Geometry check sheet. Reference: drawing and pictorial views, mm from the part's lowest x, y, z. A direction names the side the tool comes from. Coordinates: 2 decimals unless noted, no trailing zeros. Order: outer loops, then holes, each group sorted by start corner. A loop starts at its lowest first (then second) coordinate and runs counter-clockwise, first axis right, second up. Notation, with made-up numbers: M 78.25,20 L 84.25,20 A21 cw 84.25,30 Z; hole C 79.5,16.5 d10. An arc over 180 degrees is marked long. Return JSON: item names as keys, results as strings.
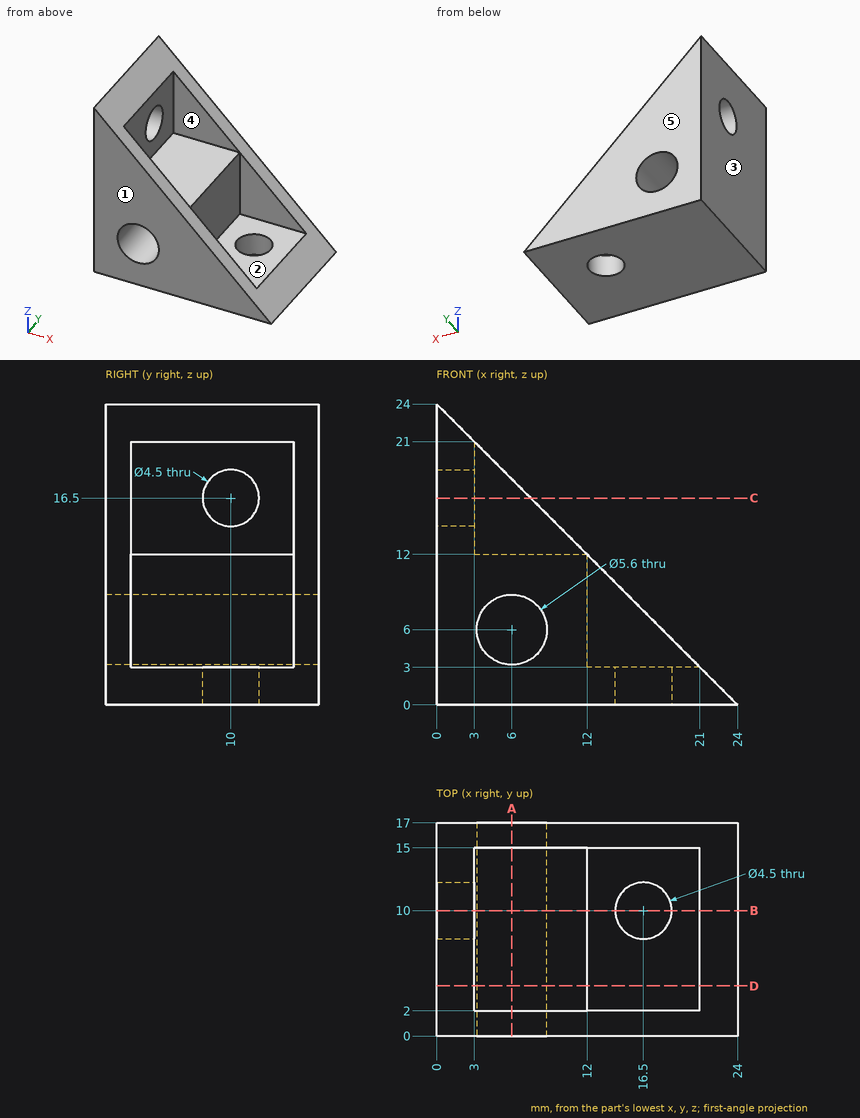
Q1. Cross-section at C-C, the plane z = 16.5. Record the boundary of the cut face in (x, y), and give its area (3 significant figures).
Values:
{"outline": "M 0,0 L 7.5,0 L 7.5,2 L 3,2 L 3,7.75 L 0,7.75 Z; M 0,12.25 L 3,12.25 L 3,15 L 7.5,15 L 7.5,17 L 0,17 Z", "area": "55.5 mm^2"}
Q2. Material ranges on line 1 along Y through (x, z) = (4, 15.5); line 2 along Y through (x, z) = (16.5, 1.4); line 3 along Z through (x, y) = (6, 5.25), recorded low to high.
Values:
{"line 1": "0 to 2, 15 to 17", "line 2": "0 to 7.75, 12.25 to 17", "line 3": "0 to 3.2, 8.8 to 12"}
Q3. Cross-section at D-D, the plane y = 4. Record the boundary of the cut face in (x, z), and give its area (3 significant figures).
Values:
{"outline": "M 0,0 L 24,0 L 21,3 L 12,3 L 12,12 L 3,12 L 3,21 L 0,24 Z; hole C 6,6 d5.6", "area": "182 mm^2"}
Q4. Cross-section at A-A, the plane x = 6. Record the boundary of the cut face in (y, z), and give its area (3 significant figures).
Values:
{"outline": "M 0,0 L 17,0 L 17,3.2 L 0,3.2 Z; M 0,8.8 L 17,8.8 L 17,18 L 15,18 L 15,12 L 2,12 L 2,18 L 0,18 Z", "area": "133 mm^2"}
Q5. Go/stop test with flat-tipped pins: pin 1 (2.5 mm diameter, centred on x = 17.5, y = 8.5, fed in from +Z); pin 2 (7 mm diameter, centred on y = 10, z = 16.5, fed in from -X); pin 3 (2 mm diameter, centred on y = 5, z = 16, fed in from +X); pin 4 (2.5 mm diameter, centred on x = 9.5, y = 9, fed in from +Z). Record where each tip stops, or that it passes through.
Values:
{"pin 1": "z = 3", "pin 2": "x = 0", "pin 3": "x = 3", "pin 4": "z = 12"}
Q6. Tool access check on the marked faces 4 and 5. Record the directions out of +Z, -Z, +X, -X, +Y, -Y that give a thin tool (end or side, any length) a straight path to the whole face; none if there is none.
Values:
{"face 4": "+Z, +X", "face 5": "+Z, -Z, +X, -X, +Y"}
Q7. Cross-section at B-B, the plane y = 10. Record the boundary of the cut face in (x, z).
Values:
{"outline": "M 0,0 L 14.25,0 L 14.25,3 L 12,3 L 12,12 L 3,12 L 3,14.25 L 0,14.25 Z; M 0,18.75 L 3,18.75 L 3,21 L 0,24 Z; M 18.75,0 L 24,0 L 21,3 L 18.75,3 Z; hole C 6,6 d5.6"}
Q8. Draft check along Y on the marked faces 1, 2 and 3. Enter one of: pulls with the +Y half, pulls with the -Y half, needs draft (parallel to the pull), parting line crosses it, or undercut.
Values:
{"face 1": "pulls with the -Y half", "face 2": "undercut", "face 3": "needs draft"}
